Geometry: final body of the model. Coordinates: model frame, mm. A direction names the side the tool comes from. Coordinates: 2 decimals unless noted, no trailing zeros. Loops run counter-clockwise (first coordinate to the right, second up) from the corner with the lowest first, then second, coordinate; pieces in that order, holes last. Notation, with made-up numbers: (11.25, -4.75) - (54.25, -4.75) arc R9 ccw to (54.25, 8.25) - close; hole circle Ø6 at (77, -8.5). An arc over 180 degrees is marked (long way). Answer in a Markdown table with one row per item.
from build123d import *

# Parameters (mm, degrees)
SKETCH_1_W          = 23.5
SKETCH_1_H          = 5.5
EXTRUDE_1_DEPTH     = 2
SKETCH_2_W          = 0.5
SKETCH_2_H          = 1
CUT_EXTRUDE_1_DEPTH = 13.232129823
SKETCH_4_W          = 2
SKETCH_4_H          = 1
EXTRUDE_2_DEPTH     = 0.2
SKETCH_5_W          = 21.5
SKETCH_5_H          = 0.2
EXTRUDE_3_DEPTH     = 0.3
SKETCH_6_W          = 21.5
SKETCH_6_H          = 0.7
CUT_EXTRUDE_2_DEPTH = 4.5
CUT_EXTRUDE_3_DEPTH = 0.002
SKETCH_8_W          = 21.5
SKETCH_8_H          = 0.5
CUT_EXTRUDE_4_DEPTH = 0.5


with BuildPart() as part:
    # 草图1 → 凸台-拉伸1 (new body)
    with BuildSketch(Plane(origin=(0, 0, 0), x_dir=(1, 0, 0), z_dir=(0, 1, 0))):
        Rectangle(SKETCH_1_W, SKETCH_1_H)
    extrude(amount=EXTRUDE_1_DEPTH)

    # 草图2 → 切除-拉伸1 (cut, through all)
    with BuildSketch(Plane(origin=(0, 2, 0), x_dir=(1, 0, 0), z_dir=(0, 1, 0))):
        with Locations((-11.5, 2.25)):
            Rectangle(SKETCH_2_W, SKETCH_2_H)
        with Locations((11.5, 2.25)):
            Rectangle(SKETCH_2_W, SKETCH_2_H)
    extrude(amount=-CUT_EXTRUDE_1_DEPTH, mode=Mode.SUBTRACT)

    # 草图4 → 凸台-拉伸2 (add)
    with BuildSketch(Plane.XZ):
        with Locations((-11.75, 1.25)):
            Rectangle(SKETCH_4_W, SKETCH_4_H)
        with Locations((11.75, 1.25)):
            Rectangle(SKETCH_4_W, SKETCH_4_H)
    extrude(amount=EXTRUDE_2_DEPTH)

    # 草图5 → 凸台-拉伸3 (add)
    with BuildSketch(Plane.XZ):
        with Locations((0, -2.45)):
            Rectangle(SKETCH_5_W, SKETCH_5_H)
    extrude(amount=EXTRUDE_3_DEPTH)

    # 草图6 → 切除-拉伸2 (cut)
    with BuildSketch(Plane.XY.offset(2.75)):
        with Locations((0, 1.35)):
            Rectangle(SKETCH_6_W, SKETCH_6_H)
    extrude(amount=-CUT_EXTRUDE_2_DEPTH, mode=Mode.SUBTRACT)

    # 草图7 → 切除-拉伸3 (cut)
    with BuildSketch(Plane(origin=(0, 2, 0), x_dir=(1, 0, 0), z_dir=(0, 1, 0))):
        Polygon((-11.25, 1.75), (-11.25, 0.773341088), (-10.75, 0.773341088), (-10.75, 1.273341088), (10.75, 1.273341088), (10.75, 0.773341088), (11.25, 0.773341088), (11.25, 1.75), (11.75, 1.75), (11.75, -2.75), (-11.75, -2.75), (-11.75, 1.75), align=None)
    extrude(amount=-CUT_EXTRUDE_3_DEPTH, mode=Mode.SUBTRACT)

    # 草图8 → 切除-拉伸4 (cut)
    with BuildSketch(Plane(origin=(0, 2, 0), x_dir=(1, 0, 0), z_dir=(0, 1, 0))):
        with Locations((0, 1.523341088)):
            Rectangle(SKETCH_8_W, SKETCH_8_H)
    extrude(amount=-CUT_EXTRUDE_4_DEPTH, mode=Mode.SUBTRACT)


solid = part.part
(1) Ray query, probe 1 along X at (y, z) = (1.35, 2.4); probe 2 along Y at (x, z) = (-8.5, 1.1); probe 3 along X at (y, z) = (-0.05, 1.35). Return the intervals inside material, ascending.
Verdict:
| item | result |
|---|---|
| probe 1 | x = -11.75 to -10.75, 10.75 to 11.75 |
| probe 2 | y = 0 to 1, 1.7 to 2 |
| probe 3 | x = -12.75 to -10.75, 10.75 to 12.75 |
(2) Cut plane D-D on z = -0.1. Output: boundary loops of the cut face in (x, y), then the cut area to 3 significant figures.
Verdict:
| item | result |
|---|---|
| outline | (-11.75, 0) - (11.75, 0) - (11.75, 2) - (-11.75, 2) - close; hole (-10.75, 1) - (10.75, 1) - (10.75, 1.7) - (-10.75, 1.7) - close |
| area | 31.9 mm² |
(3) Cut plane B-B on z = 1.05. Output: boundary loops of the cut face in (x, y), then the cut area to 3 significant figures.
Verdict:
| item | result |
|---|---|
| outline | (-12.75, -0.2) - (-10.75, -0.2) - (-10.75, 0) - (10.75, 0) - (10.75, -0.2) - (12.75, -0.2) - (12.75, 0) - (11.75, 0) - (11.75, 2) - (-11.75, 2) - (-11.75, 0) - (-12.75, 0) - close; hole (-10.75, 1) - (10.75, 1) - (10.75, 1.7) - (-10.75, 1.7) - close |
| area | 32.7 mm² |
(4) Access query for faces 4 (the face through (12, 0, 1)), 5 (the face through (0, 1, 1)), 6 (the face through (0, 1.998, 0)), 7 (the face through (-11.75, 1, 1)). Directions: +Z, -Z, +X, -X, +Y, -Y. A direction counts if a zero-diameter tool reaches every point of the face in a straight line with its end or side. Return the directions, or none.
Verdict:
| item | result |
|---|---|
| face 4 | +Z, -Z, +X, +Y |
| face 5 | +Z |
| face 6 | +Z, -Z, +X, -X, +Y |
| face 7 | +Z, -Z, -X, +Y |
(5) Pull-direction query (X, two-part tool) for faces 1 (the face through (0, 0, 1)), 2 (the face through (0, 1, -2.75)), 3 (the face through (11.25, 1, -2)); classes: pulls with the +X half, pulls with the -X half, needs draft (parallel to the pull), parting line crosses it, or undercut.
Verdict:
| item | result |
|---|---|
| face 1 | undercut |
| face 2 | needs draft |
| face 3 | pulls with the +X half |
(6) First-contact query: pin 1 Ø1.2 at (x, z) = (3.5, 1.5) entering from -Y; pin 2 Ø0.6 at (x, y) = (-2, 1.5) entering from +Z; pin 3 Ø1.1 at (x, z) = (-11.5, 1.5) entering from -Y. Flat tips, straight axial feed; report the tip coordinate or a pass-through.
Verdict:
| item | result |
|---|---|
| pin 1 | stops at y = 0 |
| pin 2 | stops at z = 2.75 |
| pin 3 | stops at y = -0.2 |
